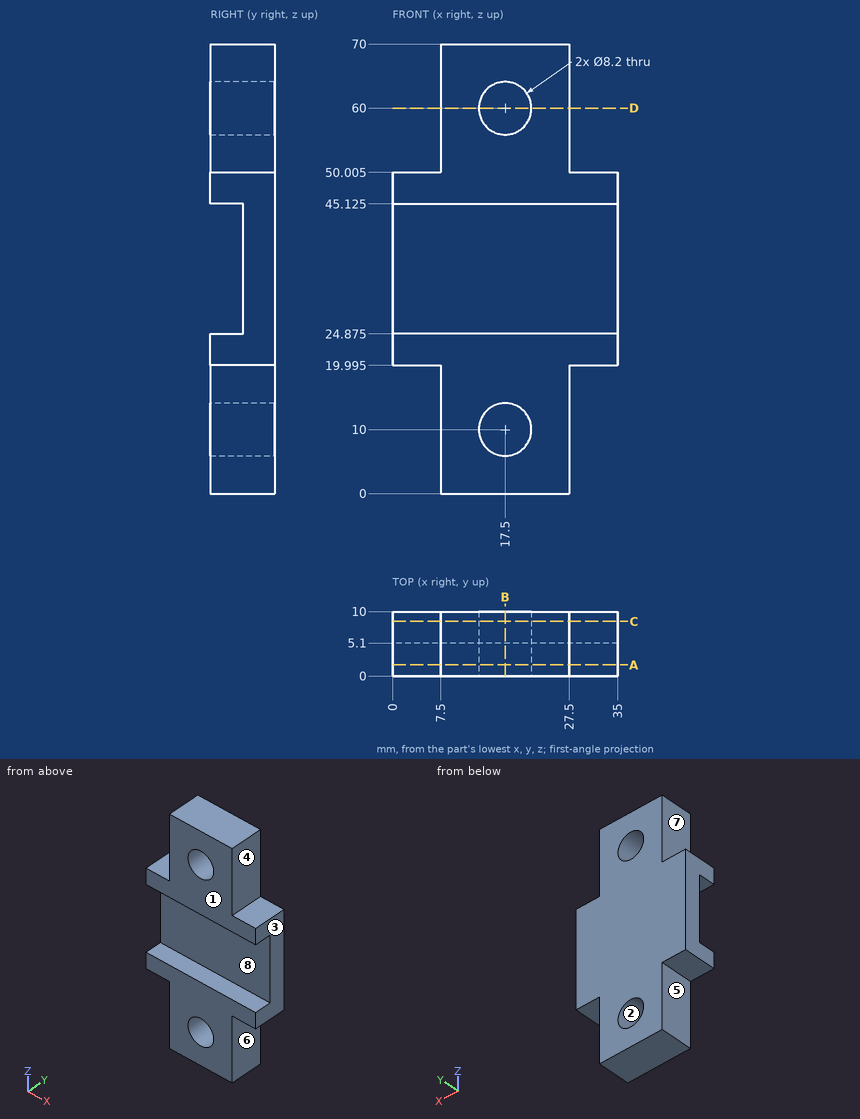
Geometry: see drawing. Coordinates: mm, zero at the bounding-box minimum. A direction names the side the tool comes from. Give positions to 0.01 mm unless a question says otherwise; leave off trailing zeros. Loops run counter-clockwise (first coordinate to the right, second up) from the corner with the lowest first, then second, coordinate; pieces in that order, holes last. Notation, with made-up numbers: (76.5, -26.75) -> (123.5, -26.75) arc R21 cw to (123.5, 9.25) -> close; hole circle Ø1 at (7.5, 5). An arc over 180 degrees is marked (long way). Answer as a JSON object with one key per item and string values. Group by question number.
Item 1: Pull-direction query (X, two-part tool) for the marked faces 1, 2 and 3; classes: released by +X, released by -X, zero draft, split by the parting line, or undercut.
Item 2: Line query: probe 1 along X at (y, z) = (6.75, 10); probe 2 along Z at (x, y) = (15, 7.25); probe 3 along Z at (x, y) = (10, 2.75) (3 decimals). Output: solid intervals per line, ascending.
Item 3: Pin query (flat end, axial travel): P1, Ø2, axis at x = 31, y = 8, coming from the +Z side (3 decimals); P2, Ø1.5, axis at y = 7, z = 18, coming from the +X side; P3, Ø5, axis at y = 2.5, z = 56.5, coming from the -X side. Return the tip coordinate at first contact, or that it passes through.
Item 4: Reachability of the marked faces 4, 5, 6, 7 and 8 from +Z, -Z, +X, -X, +Y, -Y: full face, straight path, thin tool, end or side. Return the list, or none.
Item 5: Cut plane D-D, the plane z = 60. Return the cut outline in (x, y).
Item 6: Cut plane A-A, the plane y = 1.75. Return the cut outline in (x, z) (3 decimals), and give its area (3 significant figures).
Item 7: Cut plane B-B, the plane x = 17.5. Return the cut outline in (y, z) (3 decimals), and give its area (3 significant figures).
Item 8: Cut plane C-C, the plane y = 8.5. Return the cut outline in (x, z) (3 decimals), and give its area (3 significant figures).
Checks:
{
 "1": {"face 1": "zero draft", "face 2": "undercut", "face 3": "released by +X"},
 "2": {"probe 1": "x = 7.5 to 13.4, 21.6 to 27.5", "probe 2": "z = 0 to 6.75, 13.25 to 56.75, 63.25 to 70", "probe 3": "z = 0 to 24.875, 45.125 to 70"},
 "3": {"P1": "stops at z = 50.005", "P2": "stops at x = 27.5", "P3": "stops at x = 7.5"},
 "4": {"face 4": "+Z, +X, +Y, -Y", "face 5": "-Z, -X, +Y, -Y", "face 6": "-Z, +X, +Y, -Y", "face 7": "+Z, -X, +Y, -Y", "face 8": "+X, -X, -Y"},
 "5": {"outline": "(7.5, 0) -> (13.4, 0) -> (13.4, 10) -> (7.5, 10) -> close; (21.6, 0) -> (27.5, 0) -> (27.5, 10) -> (21.6, 10) -> close"},
 "6": {"outline": "(0, 19.995) -> (7.5, 19.995) -> (7.5, 0) -> (27.5, 0) -> (27.5, 19.995) -> (35, 19.995) -> (35, 24.875) -> (0, 24.875) -> close; (0, 45.125) -> (35, 45.125) -> (35, 50.005) -> (27.5, 50.005) -> (27.5, 70) -> (7.5, 70) -> (7.5, 50.005) -> (0, 50.005) -> close; hole circle Ø8.2 at (17.5, 10); hole circle Ø8.2 at (17.5, 60)", "area": "1,040 mm²"},
 "7": {"outline": "(0, 0) -> (10, 0) -> (10, 5.9) -> (0, 5.9) -> close; (0, 14.1) -> (10, 14.1) -> (10, 55.9) -> (0, 55.9) -> (0, 45.125) -> (5.1, 45.125) -> (5.1, 24.875) -> (0, 24.875) -> close; (0, 64.1) -> (10, 64.1) -> (10, 70) -> (0, 70) -> close", "area": "433 mm²"},
 "8": {"outline": "(0, 19.995) -> (7.5, 19.995) -> (7.5, 0) -> (27.5, 0) -> (27.5, 19.995) -> (35, 19.995) -> (35, 50.005) -> (27.5, 50.005) -> (27.5, 70) -> (7.5, 70) -> (7.5, 50.005) -> (0, 50.005) -> close; hole circle Ø8.2 at (17.5, 10); hole circle Ø8.2 at (17.5, 60)", "area": "1,740 mm²"}
}
